```python
from build123d import *

# Parameters (mm, degrees)
SKETCH1_R           = 101.6
BOSS_EXTRUDE1_DEPTH = 3.175
CUT_EXTRUDE3_DEPTH  = 1.5875


with BuildPart() as part:
    # Sketch1 → Boss-Extrude1 (new body)
    with BuildSketch(Plane.XY):
        Circle(SKETCH1_R)
    extrude(amount=BOSS_EXTRUDE1_DEPTH)

    # Sketch2 → Cut-Extrude3 (cut)
    with BuildSketch(Plane(origin=(0, 0, 0), x_dir=(-1, 0, 0), z_dir=(0, 0, -1))):
        with BuildLine():
            ThreePointArc((-88.771189624, -49.418983121), (-87.988181024, -50.8), (-87.183689624, -52.168613778))
            Line((-87.183689624, -52.168613778), (-1.5875, -2.749630657))
            Line((-1.5875, -2.749630657), (-1.5875, -0.916543552))
            Line((-1.5875, -0.916543552), (-3.175, 0))
            Line((-3.175, 0), (-88.771189624, -49.418983121))
        make_face()
        Polygon((-1.5875, -0.916543552), (-1.5875, -2.749630657), (0, -1.833087105), align=None)
        Polygon((-1.5875, -0.916543552), (0, -1.833087105), (1.5875, -0.916543552), (1.5875, 0.916543552), (0, 1.833087105), (-1.5875, 0.916543552), align=None)
        Polygon((1.5875, -0.916543552), (0, -1.833087105), (1.5875, -2.749630657), align=None)
        Polygon((-3.175, 0), (-1.5875, -0.916543552), (-1.5875, 0.916543552), align=None)
        Polygon((-1.5875, 2.749630657), (-1.5875, 0.916543552), (0, 1.833087105), align=None)
        Polygon((0, 1.833087105), (1.5875, 0.916543552), (1.5875, 2.749630657), align=None)
        Polygon((1.5875, 0.916543552), (1.5875, -0.916543552), (3.175, 0), align=None)
        with BuildLine():
            Line((1.5875, 0.916543552), (3.175, 0))
            Line((3.175, 0), (88.771189624, 49.418983121))
            ThreePointArc((88.771189624, 49.418983121), (87.988181024, 50.8), (87.183689624, 52.168613778))
            Line((87.183689624, 52.168613778), (1.5875, 2.749630657))
            Line((1.5875, 2.749630657), (1.5875, 0.916543552))
        make_face()
        with BuildLine():
            Line((3.175, 0), (1.5875, -0.916543552))
            Line((1.5875, -0.916543552), (1.5875, -2.749630657))
            Line((1.5875, -2.749630657), (87.183689624, -52.168613778))
            ThreePointArc((87.183689624, -52.168613778), (87.988181024, -50.8), (88.771189624, -49.418983121))
            Line((88.771189624, -49.418983121), (3.175, 0))
        make_face()
        with BuildLine():
            Line((-1.5875, 2.749630657), (0, 1.833087105))
            Line((0, 1.833087105), (1.5875, 2.749630657))
            Line((1.5875, 2.749630657), (1.5875, 101.587596899))
            ThreePointArc((1.5875, 101.587596899), (0, 101.6), (-1.5875, 101.587596899))
            Line((-1.5875, 101.587596899), (-1.5875, 2.749630657))
        make_face()
        with BuildLine():
            Line((-88.771189624, 49.418983121), (-3.175, 0))
            Line((-3.175, 0), (-1.5875, 0.916543552))
            Line((-1.5875, 0.916543552), (-1.5875, 2.749630657))
            Line((-1.5875, 2.749630657), (-87.183689624, 52.168613778))
            ThreePointArc((-87.183689624, 52.168613778), (-87.988181024, 50.8), (-88.771189624, 49.418983121))
        make_face()
        with BuildLine():
            Line((0, -1.833087105), (-1.5875, -2.749630657))
            Line((-1.5875, -2.749630657), (-1.5875, -101.587596899))
            ThreePointArc((-1.5875, -101.587596899), (0, -101.6), (1.5875, -101.587596899))
            Line((1.5875, -101.587596899), (1.5875, -2.749630657))
            Line((1.5875, -2.749630657), (0, -1.833087105))
        make_face()
    extrude(amount=-CUT_EXTRUDE3_DEPTH, mode=Mode.SUBTRACT)


solid = part.part
```
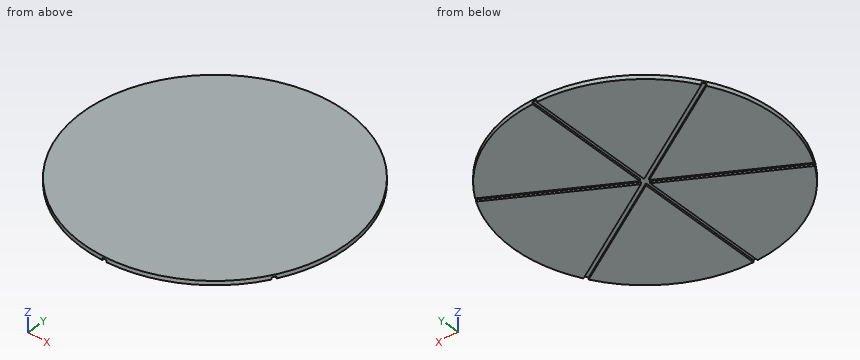
The listing builds one solid part. Answer for the finished solid, in the listing's coordinates (mm). Coordinates: 2 decimals unless noted, no trailing zeros. Write each loop counter-clockwise with the first axis right and the second up, starting at its lowest first coordinate (ties: lowest second). Pieces come first, ordered by that corner, then holes. Notation, with made-up numbers: (18, 27.25) - (59, 27.25) arc R18 cw to (59, 47.25) - close; hole circle Ø5 at (-24.5, -27). An arc over 180 degrees is marked (long way). Return JSON: item names as keys, results as strings. Group by question number.
1. Given pin 1 (0.8 mm diameter, centred on y = 46, z = 1, fed in from -X); pin 2 (1.7 mm diameter, centred on y = 33.5, z = 1, fed in from +X); pin 3 (0.5 mm diameter, centred on y = -58, z = 0.5, fed in from -X), each flat-ended and moving along its own axis, determine where each tip first touches the part or whether it passes through.
2. Straight lines are drawn through the part: L1, parallel to X at y = -21.5, z = 1; L2, parallel to Y at x = 31.5, z = 1.3; L3, parallel to X at y = -6.5, z = 0.85. For each, find the intervals that lie inside material, in ascending order.
3. A cutting plane is placed at B-B, the plane x = 35. Determine the outline of the cut face in (y, z) (1 decimal), plus the area to 3 significant figures.
4. A cutting plane is placed at A-A, the plane y = 16. Determine the outline of the cut face in (x, z) (1 decimal).
5. A cutting plane is placed at D-D, the plane y = 65.5. Determine the outline of the cut face in (x, z) (1 decimal).
6. A cutting plane is placed at C-C, the plane z = 2.45. Determine the outline of the cut face in (x, y).
Ans:
{
 "1": {"pin 1": "x = -90.79", "pin 2": "x = 96.21", "pin 3": "x = -83.59"},
 "2": {"L1": "-99.3 to -40.41, -34.06 to -1.59, 1.59 to 34.06, 40.41 to 99.3", "L2": "-96.59 to -20.02, -16.35 to 16.35, 20.02 to 96.59", "L3": "-101.39 to -14.43, -8.08 to -1.59, 1.59 to 8.08, 14.43 to 101.39"},
 "3": {"outline": "(-95.4, 0) - (-22, 0) - (-22, 1.6) - (-18.4, 1.6) - (-18.4, 0) - (18.4, 0) - (18.4, 1.6) - (22, 1.6) - (22, 0) - (95.4, 0) - (95.4, 3.2) - (-95.4, 3.2) - close", "area": "594 mm²"},
 "4": {"outline": "(-100.3, 0) - (-30.9, 0) - (-30.9, 1.6) - (-24.5, 1.6) - (-24.5, 0) - (-1.6, 0) - (-1.6, 1.6) - (1.6, 1.6) - (1.6, 0) - (24.5, 0) - (24.5, 1.6) - (30.9, 1.6) - (30.9, 0) - (100.3, 0) - (100.3, 3.2) - (-100.3, 3.2) - close"},
 "5": {"outline": "(-77.7, 0) - (-1.6, 0) - (-1.6, 1.6) - (1.6, 1.6) - (1.6, 0) - (77.7, 0) - (77.7, 3.2) - (-77.7, 3.2) - close"},
 "6": {"outline": "circle Ø203.2 at (0, 0)"}
}
